Build history of the part. All positions in model axes, mm. Face numbers are marked on the shaded views. A direction names the side the tool comes from. Give positions to 0.01 mm unless a question says otherwise; leave off trailing zeros. Order: outer loops, then holes, each group sorted by start corner. A loop starts at its lowest first (then second) coordinate and runs counter-clockwise, first axis right, second up. Notation, with made-up numbers: M 68.25,5 L 105.25,5 A19 ccw 105.25,37 Z; hole C 33.5,-23 d2. An arc over 180 degrees is marked long. Answer as CSV lines item,"result".
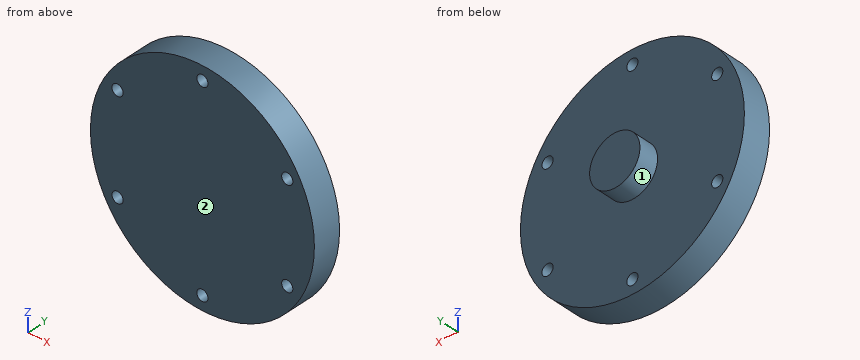
Autodesk Inventor part; units mm, degrees
ref_plane "YZ Plane" through (0, 0, 0) normal (1, 0, 0) x (0, 1, 0)
ref_plane "XZ Plane" through (0, 0, 0) normal (0, 1, 0) x (-1, 0, 0)
ref_plane "XY Plane" through (0, 0, 0) normal (0, 0, 1) x (1, 0, 0)
sketch "Sketch1" plane through (0, 0, 0) normal (0, 1, 0) x (-1, 0, 0)
  circle A0 centre (0, 0) radius 40
  line L0 (0, 40) -> (40, 40) construction
  line L1 (0, 0) -> (0, 7.8266) construction
  line L2 (0, 0) -> (7.0888, 0) construction
  dimension "d0" = 80
extrude "Extrusion1" add sketch "Sketch1" along normal blind 10
sketch "Sketch2" plane through (0, 10, 0) normal (0, 1, 0) x (1, 0, 0)
  circle A0 centre (0, 0) radius 40
  line L0 (0, -40) -> (-40, -40) construction
  line L1 (0, 0) -> (0, 3.1787) construction
  line L2 (0, 0) -> (-7.099, 0) construction
  line L3 (0, 0) -> (-40, -40)
  line L4 (0, 0) -> (40, -40)
  line L5 (0, 0) -> (-40, 40)
  line L6 (0, 0) -> (40, 40)
  circle A1 centre (0, 0) radius 40 construction
  line L7 (-28.2843, -28.2843) -> (-24.7487, -24.7487) construction
  circle A2 centre (0, 0) radius 35 construction
  circle A3 centre (-35, 0) radius 2
  circle A4 centre (-30.3109, -17.5) radius 2
  circle A5 centre (-17.5, -30.3109) radius 2
  circle A6 centre (0, -35) radius 2
  circle A7 centre (17.5, -30.3109) radius 2
  circle A8 centre (30.3109, -17.5) radius 2
  circle A9 centre (35, 0) radius 2
  circle A10 centre (30.3109, 17.5) radius 2
  circle A11 centre (17.5, 30.3109) radius 2
  circle A12 centre (0, 35) radius 2
  circle A13 centre (-17.5, 30.3109) radius 2
  circle A14 centre (-30.3109, 17.5) radius 2
  dimension "d4" = 5
  dimension "d5" = 4
  dimension "d8" = 360
extrude "Extrusion2" cut sketch "Sketch2" against normal through all contours A4 | A6 | A8 | A10 | A12 | A14
sketch "Sketch3" plane through (0, 0, 0) normal (0, -1, 0) x (1, 0, 0)
  point P0 (0, 0)
sketch "Sketch4" plane through (0, 10, 0) normal (0, 1, 0) x (1, 0, 0)
  circle A0 centre (0, 0) radius 9
  dimension "d12" = 18
extrude "Extrusion3" add sketch "Sketch4" along normal blind 7
properties part number "magnet bottom"
Item 1: Band-saw the part on D-D (z = 0). Give the cut face in (x, y).
Geometry says:
outline,"M -40,0 L 40,0 L 40,10 L 9,10 L 9,17 L -9,17 L -9,10 L -40,10 Z"
Item 2: 3-axis set-ups, long thin cutter, end or side, ignore diameter. For the marked faces 1 and 2: which of +Z, -Z, +X, -X, +Y, -Y reach the whole face in a straight line?
Geometry says:
face 1,"+Y"
face 2,"+Z, -Z, +X, -X, -Y"
Item 3: Band-saw the part on A-A (x = 0). Give the cut face in (y, z).
Geometry says:
outline,"M 0,-40 L 10,-40 L 10,-37 L 0,-37 Z; M 0,-33 L 10,-33 L 10,-9 L 17,-9 L 17,9 L 10,9 L 10,33 L 0,33 Z; M 0,37 L 10,37 L 10,40 L 0,40 Z"
Item 4: Band-saw the part on B-B (y = 3). Give the cut face in (x, z).
Geometry says:
outline,"C 0,0 d80; hole C -30.31,-17.5 d4; hole C -30.31,17.5 d4; hole C 0,-35 d4; hole C 0,35 d4; hole C 30.31,-17.5 d4; hole C 30.31,17.5 d4"
Item 5: Drop flat-ended pins along their axis: pin 1 (8 mm diameter, centred on x = 14.5, z = -5, fed in from +Y); pin 2 (2 mm diameter, centred on x = -10, y = 4.5, fed in from -Z); pin 3 (5 mm diameter, centred on y = 2, z = 25.5, fed in from -X). Give the stop position or say it passes through.
Geometry says:
pin 1,"stops at y = 10"
pin 2,"stops at z = -38.97"
pin 3,"stops at x = -32.73"
Item 6: Band-saw the part on C-C (z = -16.5). Give the cut face in (x, y).
Geometry says:
outline,"M -36.44,0 L -32.04,0 L -32.04,10 L -36.44,10 Z; M -28.58,0 L 28.58,0 L 28.58,10 L -28.58,10 Z; M 32.04,0 L 36.44,0 L 36.44,10 L 32.04,10 Z"
Item 7: Probe line 1 along Z through (x, y) = (0, 6); line 2 along X through (y, z) = (7.5, 17.5); line 3 along Z through (x, y) = (-0.5, 4.5). List the from-to ranges inside material, lowest first. Write a range as from..to.
Geometry says:
line 1,"z = -40..-37, -33..33, 37..40"
line 2,"x = -35.97..-32.31, -28.31..28.31, 32.31..35.97"
line 3,"z = -40..-36.94, -33.06..33.06, 36.94..40"
